Geometry: final body of the model. Coordinates: model frame, mm. Coordinates: 2 decimals unless noted, no trailing zeros. Loops run counter-clockwise (first coordinate to the right, second up) from the corner with the lowest first, then second, coordinate; pieces in that order, holes last. Notation, with made-up numbers: (2, -17) -> (47, -17) arc R31 ccw to (47, 11) -> close; hole circle Ø5 at (57.5, -29.75). An arc over 180 degrees is marked (long way). One line per item, written item: value. Start each with the question number.
from build123d import *

# Parameters (mm, degrees)
SKETCH1_W           = 25.4
SKETCH1_H           = 3.302
BOSS_EXTRUDE1_DEPTH = 3.302


with BuildPart() as part:
    # Sketch1 → Boss-Extrude1 (new body)
    # profile 1 of 2: a face of its own
    with BuildSketch(Plane(origin=(0, 0, 0), x_dir=(1, 0, 0), z_dir=(0, 1, 0))):
        with BuildLine():
            Line((12.7, -3.302), (12.7, 0))
            Line((12.7, 0), (36.3474, 0))
            Line((36.3474, 0), (36.3474, 3.175))
            Line((36.3474, 3.175), (33.3375, 3.175))
            Line((33.3375, 3.175), (33.3375, 6.35))
            Line((33.3375, 6.35), (36.3474, 6.35))
            Line((36.3474, 6.35), (36.3474, 9.525))
            Line((36.3474, 9.525), (39.8526, 9.525))
            Line((39.8526, 9.525), (39.8526, 6.35))
            Line((39.8526, 6.35), (42.8625, 6.35))
            Line((42.8625, 6.35), (42.8625, 3.175))
            Line((42.8625, 3.175), (39.8526, 3.175))
            Line((39.8526, 3.175), (39.8526, 0))
            Line((39.8526, 0), (66.675, 0))
            Line((66.675, 0), (92.075, 0))
            Line((92.075, 0), (118.8974, 0))
            Line((118.8974, 0), (118.8974, 3.175))
            Line((118.8974, 3.175), (115.8875, 3.175))
            Line((115.8875, 3.175), (115.8875, 6.35))
            Line((115.8875, 6.35), (118.8974, 6.35))
            Line((118.8974, 6.35), (118.8974, 9.525))
            Line((118.8974, 9.525), (122.4026, 9.525))
            Line((122.4026, 9.525), (122.4026, 6.35))
            Line((122.4026, 6.35), (125.4125, 6.35))
            Line((125.4125, 6.35), (125.4125, 3.175))
            Line((125.4125, 3.175), (122.4026, 3.175))
            Line((122.4026, 3.175), (122.4026, 0))
            Line((122.4026, 0), (146.05, 0))
            Line((146.05, 0), (146.05, -3.302))
            Line((146.05, -3.302), (158.75, -3.302))
            Line((158.75, -3.302), (158.75, 9.398))
            Line((158.75, 9.398), (56.528812184, 131.220467819))
            ThreePointArc((56.528812184, 131.220467819), (12.697978408, 72.316136438), (0, 0))
            Line((0, 0), (0, -3.302))
            Line((0, -3.302), (12.7, -3.302))
        make_face()
        with BuildLine():
            ThreePointArc((145.652391105, 13.177751924), (144.994827074, 14.765251924), (145.652391105, 16.352751924))
            ThreePointArc((145.652391105, 16.352751924), (147.239891105, 17.010315954), (148.827391105, 16.352751924))
            ThreePointArc((148.827391105, 16.352751924), (149.314059811, 15.624400733), (149.484955135, 14.765251924))
            ThreePointArc((149.484955135, 14.765251924), (149.314059811, 13.906103115), (148.827391105, 13.177751924))
            ThreePointArc((148.827391105, 13.177751924), (147.239891105, 12.520187894), (145.652391105, 13.177751924))
        make_face(mode=Mode.SUBTRACT)
        with BuildLine():
            Line((13.889891105, 14.765251924), (10.384691105, 14.765251924))
            ThreePointArc((10.384691105, 14.765251924), (23.206957648, 72.602758658), (59.271064223, 119.602417396))
            Line((59.271064223, 119.602417396), (61.524163353, 116.917278414))
            ThreePointArc((61.524163353, 116.917278414), (26.383747703, 71.121397127), (13.889891105, 14.765251924))
        make_face(mode=Mode.SUBTRACT)
    # profile 2 of 2: a face of its own
    with BuildSketch(Plane(origin=(0, 0, 0), x_dir=(1, 0, 0), z_dir=(0, 1, 0))):
        with Locations((79.375, -1.651)):
            Rectangle(SKETCH1_W, SKETCH1_H)
    extrude(amount=BOSS_EXTRUDE1_DEPTH)


solid = part.part
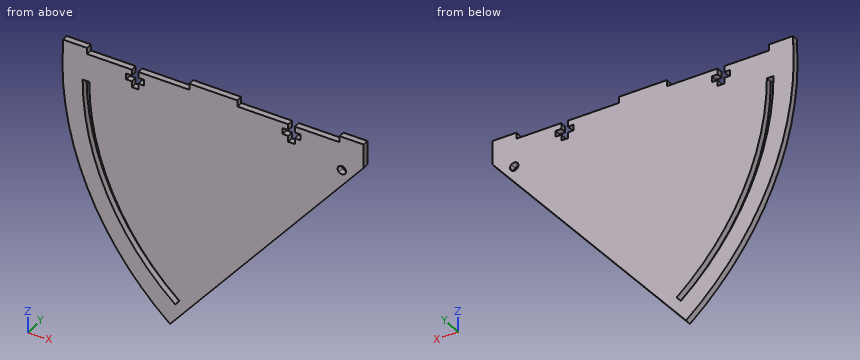
1. Line query: L1, parallel to X at y = 3, z = -5.5; L2, parallel to X at y = 1.1, z = -40; L3, parallel to Z at x = 33.5, y = 1.6 (3 decimals). Output: solid intervals per line, ascending. Write a range as [from, to].
2. Section C-C on z = -93.5. Return the cut outline in (x, y), plus the area to 3 significant figures.
3. Section A-A on z = -30. Return the cut outline in (x, y), plus the area to 3 significant figures.
4. Pin query (flat end, axial travel): pin 1 Ø0.9 at (x, y) = (117.5, 2) entering from -Z; pin 2 Ø1 at (y, z) = (1, 1) entering from -X; pin 3 Ø1.5 at (x, y) = (123.5, 1) entering from +Z; pin 4 Ø1 at (x, z) = (60.5, -51.5) entering from -Y. Return the tip coordinate at first contact, or that it passes through.
5. Section B-B on y = 1.45. Count the separate pieces of the cut face and the enclosed holes in it, plus the area to 3 significant figures.
6. Section D-D on x = 85.5. Return the cut outline in (y, z), plus the area to 3 significant figures.
Checks:
1. L1: [-0.23, 33.34], [42.86, 115.89], [125.41, 158.75]
1. L2: [2.69, 12.73], [16.3, 133.07]
1. L3: [-107.389, -90.874], [-84.375, -6.35], [-3.175, 0]
2. outline: (23.78, 0) -> (35.3, 0) -> (35.3, 3.3) -> (23.78, 3.3) -> close; (39.62, 0) -> (88.18, 0) -> (88.18, 3.3) -> (39.62, 3.3) -> close
2. area: 198 mm²
3. outline: (1.06, 0) -> (11.24, 0) -> (11.24, 3.3) -> (1.06, 3.3) -> close; (14.76, 0) -> (141.46, 0) -> (141.46, 3.3) -> (14.76, 3.3) -> close
3. area: 452 mm²
4. pin 1: z = -59.09
4. pin 2: x = 0
4. pin 3: z = 0
4. pin 4: y = 0
5. separate pieces: 1
5. enclosed holes: 2
5. area: 12,200 mm²
6. outline: (0, -96.69) -> (3.3, -96.69) -> (3.3, 3.3) -> (0, 3.3) -> close
6. area: 330 mm²
